Check sheet for the modelled part. Datum: model origin and axes. Units: mm. A direction names the side the tool comes from. Give positions to 0.01 mm unless a question says otherwise; leave off trailing zeros. Order: outer loops, then holes, each group sorted by start corner. A loop starts at its lowest first (then second) coordinate and runs counter-clockwise, first axis right, second up.
from build123d import *

# Parameters (mm, degrees)
SKETCH_W     = 33
SKETCH_H     = 10
PAD_DEPTH    = 3
SKETCH001_W  = 9
SKETCH001_H  = 10
PAD001_DEPTH = 8


with BuildPart() as part:
    # Sketch → Pad (new body)
    with BuildSketch(Plane.XY):
        Rectangle(SKETCH_W, SKETCH_H)
    extrude(amount=PAD_DEPTH)

    # Sketch001 → Pad001 (join)
    with BuildSketch(Plane.XY.offset(3)):
        with Locations((12, 0)):
            Rectangle(SKETCH001_W, SKETCH001_H)
    extrude(amount=PAD001_DEPTH)


solid = part.part
1) Set-up check for faces 1 (the face through (3, -5, 2)), 2 (the face through (-5, 0, 3)): record each of +Z, -Z, +X, -X, +Y, -Y from which the full face is reachable in a straight line by a thin tool's end or side.
Recorded:
face 1: +Z, -Z, +X, -X, -Y
face 2: +Z, -X, +Y, -Y
2) Material ranges on L1, parallel to Z at x = 3, y = 4.75; L2, parallel to X at y = 1.25, z = 6.75, recorded low to high.
Recorded:
L1: z = 0 to 3
L2: x = 7.5 to 16.5
3) Section check B-B, the plane x = 3.5. Record the cut outline in (y, z).
Recorded:
outline: (-5, 0) - (5, 0) - (5, 3) - (-5, 3) - close
4) Section check C-C, the plane y = 1.25. Record the cut outline in (x, z), then the cut area to 3 significant figures.
Recorded:
outline: (-16.5, 0) - (16.5, 0) - (16.5, 11) - (7.5, 11) - (7.5, 3) - (-16.5, 3) - close
area: 171 mm2
5) Section check A-A, the plane z = 4.5. Record the cut outline in (x, y).
Recorded:
outline: (7.5, -5) - (16.5, -5) - (16.5, 5) - (7.5, 5) - close
